from build123d import *

# Parameters (mm, degrees)
F1_DEPTH = 2414
F3_DEPTH = 29.001


with BuildPart() as f1:
    # F0 (on Top) → F1 (new body)
    with BuildSketch(Plane.XY):
        Polygon((0, 4), (0, 0), (103.747326, 0), (139.747326, -25), (411, -25), (411, -21), (141, -21), (105, 4), align=None)
    extrude(amount=F1_DEPTH)

    # F2 (on face) → F3 (cut, through all)
    with BuildSketch(Plane.XZ.offset(25)):
        Polygon((103.747326, 2414), (0, 2414), (0, 2264), (124, 2264), (124, 2414), align=None)
        Polygon((103.747326, 0), (124, 0), (124, 150), (0, 150), (0, 0), align=None)
    extrude(amount=-F3_DEPTH, mode=Mode.SUBTRACT)


solid = f1.part
Geometry: final body of the model. Coordinates: model frame, mm. A direction names the side the tool comes from. Coordinates: 2 decimals unless noted, no trailing zeros. Loops run counter-clockwise (first coordinate to the right, second up) from the corner with the lowest first, then second, coordinate; pieces in that order, holes last. Notation, with made-up numbers: M 18.25,-2.5 L 46.25,-2.5 A21 cw 46.25,31.5 Z; hole C -32.5,20 d9. An arc over 180 degrees is marked long. One line per item, written item: value. Start each with the question number.
1) Pin query (flat end, axial travel): P1, Ø5.5, axis at y = -12.5, z = 2302.5, coming from the -X side; P2, Ø1, axis at y = -9, z = 943, coming from the -X side; P3, Ø5.5, axis at x = 48.5, y = -1.5, coming from the -Z side. Return the tip coordinate at first contact, or that it passes through.
2) Cut plane B-B (x = 222.5). Return loops of the section in (y, z).
3) Reachability of faces 1 (the flat face through (278, -21, 1190)), 2 (the flat face through (51, 0, 1192)), 3 (the flat face through (273, -25, 1190)) from +Z, -Z, +X, -X, +Y, -Y: full face, straight path, thin tool, end or side. Return the list, or none.
4) Material intervals for L1, parallel to Y at x = 330, z = 2241.5; L2, parallel to Y at x = 55, z = 1707.5; L3, parallel to X at y = 0.75, z = 776, sorted ascending. Write a range as from..to.
5) Cut plane A-A (z = 1474). Return loops of the section in (x, y).
Evaluation:
1. P1: x = 124
1. P2: x = 115.99
1. P3: z = 150
2. outline: M -25,0 L -21,0 L -21,2414 L -25,2414 Z
3. face 1: +Z, -Z, +X, +Y
3. face 2: +Z, -Z, -X, -Y
3. face 3: +Z, -Z, +X, -X, -Y
4. L1: -25..-21
4. L2: 0..4
4. L3: 0..109.68
5. outline: M 0,0 L 103.75,0 L 139.75,-25 L 411,-25 L 411,-21 L 141,-21 L 105,4 L 0,4 Z
